Could you check a few things on this drawing? It's one solid part, dimensions in mm from its lowest x, y, z. A direction names the side the tool comes from. Give positions to 0.01 mm unless a question says otherwise; leave off trailing zeros. Write each loop counter-clockwise with the first axis right and the second up, starting at its lowest first coordinate (ties: lowest second). Pieces come first, ordered by that corner, then holes. Notation, with made-up numbers: M 72.25,41.25 L 100.25,41.25 A21 ccw 100.25,72.25 Z; hole C 57,-24 d4. An arc over 180 degrees is marked long. Write each question's results on one line, items separated by ' | '. Start each with the question number.
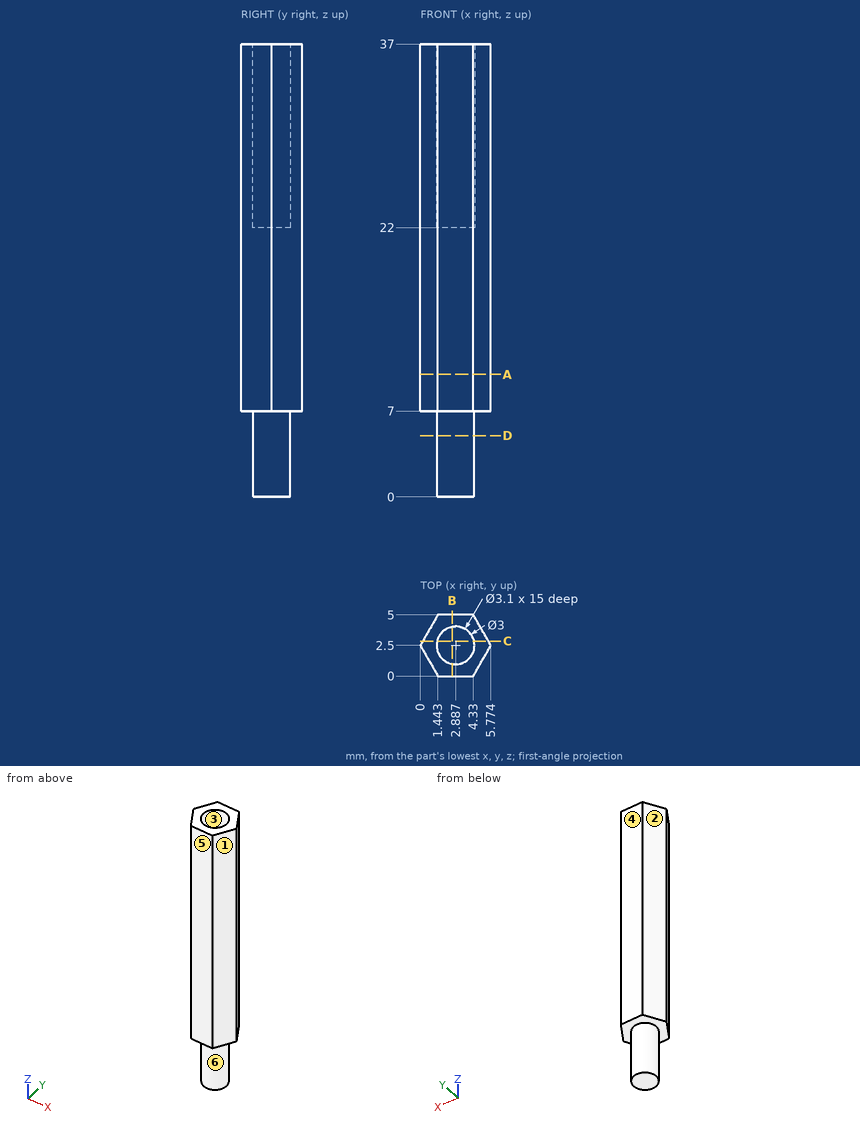
Q1. If we mould it in two halves opening along X, with no side actions, what happens to the marked faces 1, 2, 3 and 4? For each: pulls with the +X half, pulls with the -X half, needs draft (parallel to the pull), parting line crosses it, or undercut.
Q2. If we section it at B-B (x = 2.6): Please give me the cut outline in (y, z).
Q3. I'm going to push flat-ended pins straight in: P1, Ø1.5, axis at y = 2, z = 32.5, coming from the +X side; P2, Ø3, axis at y = 2.5, z = 23, coming from the -X side. Where does each tip first touch, or does it pass through?
Q4. For the marked faces 5 and 6, which set-ups out of +Z, -Z, +X, -X, +Y, -Y let a thin tool reach every point of the face, with its end or its side?
Q5. If we section it at D-D (z = 5): Please give me the cut outline in (x, y).
Q6. If we section it at C-C (y = 2.85): Please give me the cut outline in (x, z) (1 decimal).
Q7. Please list where these lines run through material, in increasing order: line 1 (Y direction, x = 3.25, z = 26); line 2 (Z direction, x = 4.55, y = 1.8); line 3 (X direction, y = 3.1, z = 31) (1 decimal). Write a range as [from, to].
Q8. If we section it at A-A (z = 10): Please give me the cut outline in (x, y).
Determined:
1) face 1: pulls with the +X half | face 2: pulls with the -X half | face 3: undercut | face 4: needs draft
2) outline: M 0,7 L 1.03,7 L 1.03,0 L 3.97,0 L 3.97,7 L 5,7 L 5,37 L 4.02,37 L 4.02,22 L 0.98,22 L 0.98,37 L 0,37 Z
3) P1: stops at x = 5.77 | P2: stops at x = 0
4) face 5: +Z, -Z, +X, -X, -Y | face 6: -Z
5) outline: C 2.89,2.5 d3
6) outline: M 0.2,7 L 1.4,7 L 1.4,0 L 4.3,0 L 4.3,7 L 5.6,7 L 5.6,37 L 4.4,37 L 4.4,22 L 1.4,22 L 1.4,37 L 0.2,37 Z
7) line 1: y = [0, 0.99], [4.01, 5] | line 2: z = [7, 37] | line 3: x = [0.3, 1.5], [4.3, 5.4]
8) outline: M 0,2.5 L 1.44,0 L 4.33,0 L 5.77,2.5 L 4.33,5 L 1.44,5 Z
